Model file for the job. Use its own axes, mm. Round coordinates to 2 decimals unless told otherwise and drop trailing zeros. Loops run counter-clockwise (first coordinate to the right, second up) from the corner with the lowest first, then second, coordinate; pieces in that order, holes last. Notation, with made-up numbers: (31, 54) -> (88, 54) arc R6 ccw to (88, 59) -> close; hole circle Ø8 at (-27, 50.25). An arc over 180 degrees is marked (long way). Use a Markdown table: item, result.
from build123d import *

# Parameters (mm, degrees)
SKETCH1_R           = 4
SKETCH1_R_2         = 3.25
SKETCH1_R_3         = 4.5
BOSS_EXTRUDE1_DEPTH = 10


with BuildPart() as part:
    # Sketch1 → Boss-Extrude1 (new body)
    with BuildSketch(Plane.XY):
        Polygon((-75, -43.301270189), (0, -86.602540378), (75, -43.301270189), (75, 43.301270189), (0, 86.602540378), (-75, 43.301270189), align=None)
        with Locations((-32.5, -56.291651246)):
            Circle(SKETCH1_R, mode=Mode.SUBTRACT)
        with Locations((-64.951905284, -37.5)):
            Circle(SKETCH1_R_2, mode=Mode.SUBTRACT)
        with Locations((-50, -29)):
            Circle(SKETCH1_R_3, mode=Mode.SUBTRACT)
        with Locations((-65, 0)):
            Circle(SKETCH1_R, mode=Mode.SUBTRACT)
        with Locations((-25, -43.301270189)):
            Circle(SKETCH1_R_3, mode=Mode.SUBTRACT)
        with Locations((-0.179491924, -40.310889132)):
            Circle(SKETCH1_R_3, mode=Mode.SUBTRACT)
        with Locations((-17.5, -30.310889132)):
            Circle(SKETCH1_R_3, mode=Mode.SUBTRACT)
        with Locations((-0.040707856, -23.070508076)):
            Circle(SKETCH1_R_3, mode=Mode.SUBTRACT)
        with Locations((-35, -20)):
            Circle(SKETCH1_R_3, mode=Mode.SUBTRACT)
        with Locations((-20, -11.5)):
            Circle(SKETCH1_R_3, mode=Mode.SUBTRACT)
        with Locations((-10, -17.320508076)):
            Circle(SKETCH1_R_3, mode=Mode.SUBTRACT)
        with Locations((0, -75)):
            Circle(SKETCH1_R_2, mode=Mode.SUBTRACT)
        with Locations((0.11473671, -57.801270189)):
            Circle(SKETCH1_R_3, mode=Mode.SUBTRACT)
        with Locations((32.5, -56.291651246)):
            Circle(SKETCH1_R, mode=Mode.SUBTRACT)
        with Locations((25, -43.301270189)):
            Circle(SKETCH1_R_3, mode=Mode.SUBTRACT)
        with Locations((17.5, -30.310889132)):
            Circle(SKETCH1_R_3, mode=Mode.SUBTRACT)
        with Locations((10, -17.320508076)):
            Circle(SKETCH1_R_3, mode=Mode.SUBTRACT)
        with BuildLine():
            ThreePointArc((16.082691215, -9.285346102), (21.145013203, -7.148110208), (24.5, -11.5))
            ThreePointArc((24.5, -11.5), (24.341353716, -12.684334375), (23.876600928, -13.785161973))
            ThreePointArc((23.876600928, -13.785161973), (17.709292144, -15.467622393), (16.082691215, -9.285346102))
        make_face(mode=Mode.SUBTRACT)
        with BuildLine():
            ThreePointArc((31.016241071, -17.907235132), (36.077748769, -15.630966058), (39.5, -20))
            ThreePointArc((39.5, -20), (39.322568769, -21.251159158), (38.804267005, -22.403654001))
            ThreePointArc((38.804267005, -22.403654001), (32.570508076, -24.208003449), (31.016241071, -17.907235132))
        make_face(mode=Mode.SUBTRACT)
        with BuildLine():
            ThreePointArc((53.95321571, -31.149903614), (47.75, -32.897114317), (46.161521, -26.651366575))
            ThreePointArc((46.161521, -26.651366575), (51.223909668, -24.440108034), (54.61473671, -28.801270189))
            ThreePointArc((54.61473671, -28.801270189), (54.446200406, -30.021279308), (53.95321571, -31.149903614))
        make_face(mode=Mode.SUBTRACT)
        with Locations((64.951905284, -37.5)):
            Circle(SKETCH1_R_2, mode=Mode.SUBTRACT)
        with Locations((-50, 0)):
            Circle(SKETCH1_R_3, mode=Mode.SUBTRACT)
        with Locations((-64.951905284, 37.5)):
            Circle(SKETCH1_R_2, mode=Mode.SUBTRACT)
        with Locations((-50.11473671, 28.801270189)):
            Circle(SKETCH1_R_3, mode=Mode.SUBTRACT)
        with Locations((-35, 0)):
            Circle(SKETCH1_R_3, mode=Mode.SUBTRACT)
        with Locations((-20, 0)):
            Circle(SKETCH1_R_3, mode=Mode.SUBTRACT)
        with Locations((-34.820508076, 20.310889132)):
            Circle(SKETCH1_R_3, mode=Mode.SUBTRACT)
        with Locations((-19.959292144, 11.570508076)):
            Circle(SKETCH1_R_3, mode=Mode.SUBTRACT)
        with Locations((-10, 17.320508076)):
            Circle(SKETCH1_R_3, mode=Mode.SUBTRACT)
        with Locations((-17.5, 30.310889132)):
            Circle(SKETCH1_R_3, mode=Mode.SUBTRACT)
        with Locations((-25, 43.301270189)):
            Circle(SKETCH1_R_3, mode=Mode.SUBTRACT)
        with Locations((-32.5, 56.291651246)):
            Circle(SKETCH1_R, mode=Mode.SUBTRACT)
        with Locations((-0.11473671, 57.801270189)):
            Circle(SKETCH1_R_3, mode=Mode.SUBTRACT)
        Circle(SKETCH1_R_3, mode=Mode.SUBTRACT)
        with Locations((10, 17.320508076)):
            Circle(SKETCH1_R_3, mode=Mode.SUBTRACT)
        with Locations((20, 0)):
            Circle(SKETCH1_R_3, mode=Mode.SUBTRACT)
        with Locations((35, 0)):
            Circle(SKETCH1_R_3, mode=Mode.SUBTRACT)
        with Locations((20, 11.5)):
            Circle(SKETCH1_R_3, mode=Mode.SUBTRACT)
        with Locations((35, 20)):
            Circle(SKETCH1_R_3, mode=Mode.SUBTRACT)
        with Locations((0.040707856, 23.070508076)):
            Circle(SKETCH1_R_3, mode=Mode.SUBTRACT)
        with Locations((17.5, 30.310889132)):
            Circle(SKETCH1_R_3, mode=Mode.SUBTRACT)
        with Locations((0.179491924, 40.310889132)):
            Circle(SKETCH1_R_3, mode=Mode.SUBTRACT)
        with Locations((25, 43.301270189)):
            Circle(SKETCH1_R_3, mode=Mode.SUBTRACT)
        with Locations((50, 0)):
            Circle(SKETCH1_R_3, mode=Mode.SUBTRACT)
        with Locations((65, 0)):
            Circle(SKETCH1_R, mode=Mode.SUBTRACT)
        with Locations((50, 29)):
            Circle(SKETCH1_R_3, mode=Mode.SUBTRACT)
        with Locations((64.951905284, 37.5)):
            Circle(SKETCH1_R_2, mode=Mode.SUBTRACT)
        with Locations((32.5, 56.291651246)):
            Circle(SKETCH1_R, mode=Mode.SUBTRACT)
        with Locations((0, 75)):
            Circle(SKETCH1_R_2, mode=Mode.SUBTRACT)
    extrude(amount=BOSS_EXTRUDE1_DEPTH)


solid = part.part
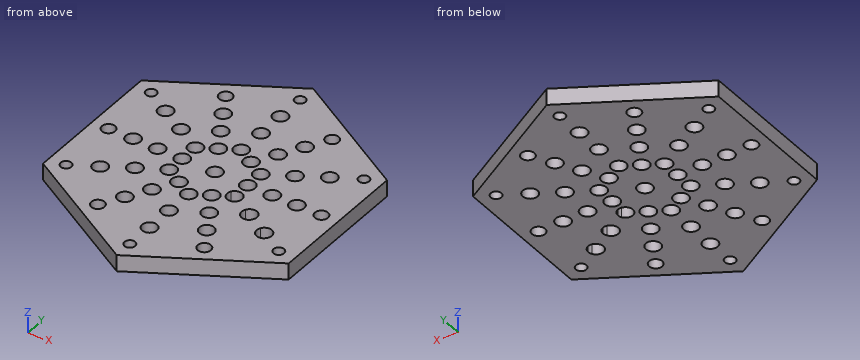
Q1. Flat gauge pins, fed straight in: pin 1 (3 mm diameter, centred on x = 35, z = 8.5, fed in from -Y); pin 2 (2 mm diameter, centred on x = 6, z = 4, fed in from -Y); pin 3 (5 mm diameter, centred on x = -11, z = 2, fed in from -Y). Where does each tip first touch, or does it go through?
Results list:
| item | result |
|---|---|
| pin 1 | stops at y = -67.26 |
| pin 2 | stops at y = -83.72 |
| pin 3 | stops at y = -81.7 |
Q2. Band-saw the part on C-C, the plane x = -65. Give the cut face in (y, z), plus the area to 3 significant figures.
Results list:
| item | result |
|---|---|
| outline | (-49.07, 0) -> (-40.75, 0) -> (-40.75, 10) -> (-49.07, 10) -> close; (-34.25, 0) -> (-4, 0) -> (-4, 10) -> (-34.25, 10) -> close; (4, 0) -> (34.25, 0) -> (34.25, 10) -> (4, 10) -> close; (40.75, 0) -> (49.07, 0) -> (49.07, 10) -> (40.75, 10) -> close |
| area | 772 mm² |
Q3. Band-saw the part on B-B, the plane y = -75. Give the cut face in (x, z), plus the area to 3 significant figures.
Results list:
| item | result |
|---|---|
| outline | (-20.1, 0) -> (-3.25, 0) -> (-3.25, 10) -> (-20.1, 10) -> close; (3.25, 0) -> (20.1, 0) -> (20.1, 10) -> (3.25, 10) -> close |
| area | 337 mm² |
Q4. Drill centre lines: L1, parallel to Y at x = 64, z = 9; L2, parallel to Y at x = -19.5, z = 5.5; L3, parallel to X at y = -28.5, z = 4.25. Where is each one in solid material? Low to high. Write a range as from..to.
Results list:
| item | result |
|---|---|
| L1 | y = -49.65..-40.61, -34.39..-3.87, 3.87..34.39, 40.61..49.65 |
| L2 | y = -75.34..-34.34, -26.28..-15.97, -7.03..-4.47, 4.47..7.09, 16.05..26.28, 34.34..75.34 |
| L3 | x = -75..-54.47, -45.53..-21.62, -13.38..13.38, 21.62..45.53, 54.6..75 |
Q5. Band-saw the part on D-D, the plane z = 5.25. Give the number of separate pieces and of enclosed holes in the cut face, plus the area to 3 significant figures.
Results list:
| item | result |
|---|---|
| separate pieces | 1 |
| enclosed holes | 49 |
| area | 16,600 mm² |
Q6. Band-saw the part on A-A, the plane x = -32.5. Give the cut face in (y, z), plus the area to 3 significant figures.
Results list:
| item | result |
|---|---|
| outline | (-67.84, 0) -> (-60.29, 0) -> (-60.29, 10) -> (-67.84, 10) -> close; (-52.29, 0) -> (-23.74, 0) -> (-23.74, 10) -> (-52.29, 10) -> close; (-16.26, 0) -> (-3.74, 0) -> (-3.74, 10) -> (-16.26, 10) -> close; (3.74, 0) -> (16.46, 0) -> (16.46, 10) -> (3.74, 10) -> close; (24.17, 0) -> (52.29, 0) -> (52.29, 10) -> (24.17, 10) -> close; (60.29, 0) -> (67.84, 0) -> (67.84, 10) -> (60.29, 10) -> close |
| area | 970 mm² |
